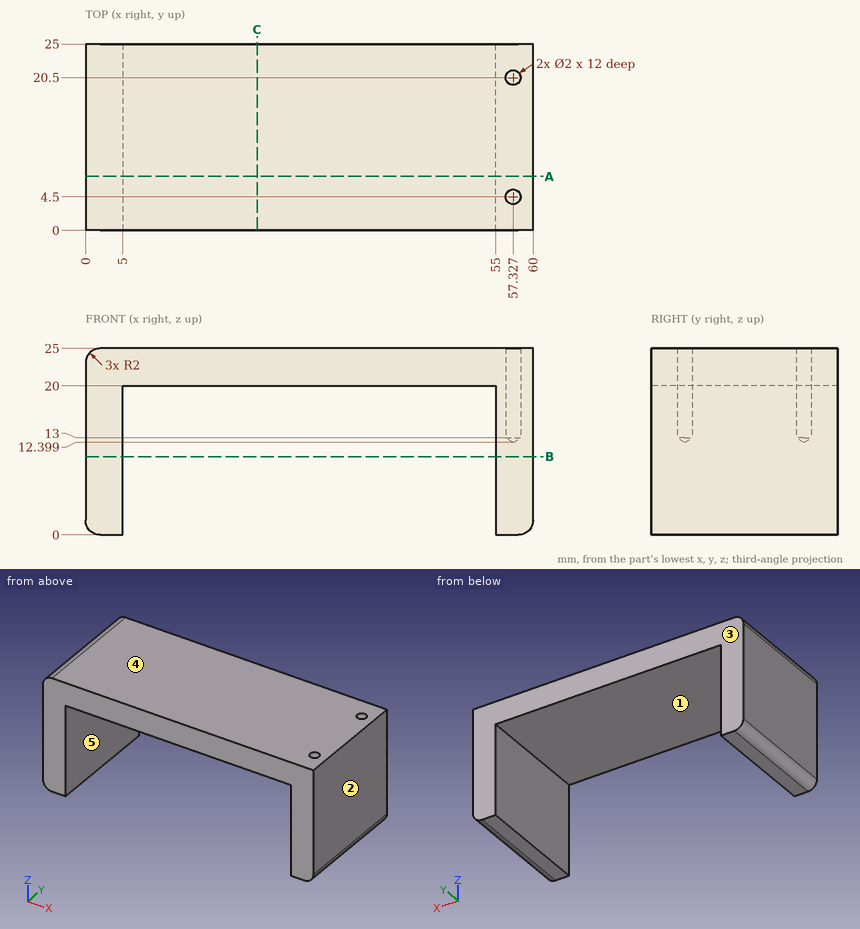
The figure shows three views and two pictorial views of one solid part (mm, origin at its lowest corner). Answer the questions. A direction names the side the tool comes from. Round coordinates to 2 decimals unless told otherwise and drop trailing zeros. Loops run counter-clockwise (first coordinate to the right, second up) from the corner with the lowest first, then second, coordinate; pieces in that order, holes last. Notation, with made-up numbers: M 0.25,2.25 L 5.25,2.25 A35 cw 5.25,36.25 Z; hole C -36.5,28.5 d4. An arc over 180 degrees is marked long. Return JSON: item names as keys, results as strings.
Q1. Find section C-C, the plane x = 23. Determine the outline of the cut face in (y, z).
Results list:
{"outline": "M 0,20 L 25,20 L 25,25 L 0,25 Z"}
Q2. The mould has two halves that part along X. Classify the marked faces 1, 2 and 3: released by +X, released by -X, zero draft, split by the parting line, or undercut.
Results list:
{"face 1": "undercut", "face 2": "released by +X", "face 3": "zero draft"}
Q3. Find the intervals of material crossed by line 1 along X through (y, z) = (4.5, 17.75); line 2 along X through (y, z) = (8.75, 12.5); line 3 along X through (y, z) = (4.5, 22.25), in increasing order. Write a range as from..to.
Results list:
{"line 1": "x = 0..5, 55..56.33, 58.33..60", "line 2": "x = 0..5, 55..60", "line 3": "x = 0..56.33, 58.33..60"}
Q4. Which of the six approach directions +Z, -Z, +X, -X, +Y, -Y give full straight-line access (tool end or side, diameter ignored) to the marked faces 4 and 5?
Results list:
{"face 4": "+Z, +X, -X, +Y, -Y", "face 5": "-Z, +Y, -Y"}
Q5. Each of these flat-tipped pins is pushed along its axis until it touches: pin 1 Ø3 at (x, y) = (47, 21) entering from -Z; pin 2 Ø10 at (y, z) = (19, 9) entering from -X. Where does it stop, or does it pass through?
Results list:
{"pin 1": "stops at z = 20", "pin 2": "stops at x = 0"}
Q6. Find section A-A, the plane y = 7.25. Determine the outline of the cut face in (x, z).
Results list:
{"outline": "M 0,2 A2 ccw 2,0 L 5,0 L 5,20 L 55,20 L 55,0 L 58,0 A2 ccw 60,2 L 60,25 L 2,25 A2 ccw 0,23 Z"}
Q7. Find section B-B, the plane z = 10.5. Determine the outline of the cut face in (x, y).
Results list:
{"outline": "M 0,0 L 5,0 L 5,25 L 0,25 Z; M 55,0 L 60,0 L 60,25 L 55,25 Z"}
